Verification items for the finished model (mm, model axes). Round coordinates to 2 decimals unless told otherwise and drop trailing zeros. Order: outer loops, then holes, each group sorted by start corner. A loop starts at its lowest first (then second) coordinate and runs counter-clockwise, first axis right, second up. Notation, with made-up numbers: M -38.5,44.5 L 2.5,44.5 A20 ccw 2.5,74.5 Z; hole C -28,45.5 d9. An arc over 180 degrees is marked long. Use one line per item in the form item = value. Start each with the question number.
Item 1: Thickness scan on probe 1 along Y at (x, z) = (-61, 38.75); probe 2 along X at (y, z) = (-24.5, 45.25); probe 3 along Y at (x, z) = (-42, 39.5). Record the ranges inside material, lowest first. Write a range as [from, to].
Item 2: Release check for a two-part mould opening along X. For faces 1 (the flat face through (-12, 0, 42)), 2 (the flat face through (64.994, -50, 42)), 3 (the cylindrical face through (-23.12, -98.48, 42.16)), 4 (the cylindrical face through (-56.414, -96.911, 42.164)) record: +X half, -X half, draft (parallel to the pull), parting line (faces both ways), or undercut.
Item 3: Cross-section at B-B on y = -21.5. Enter the section's corners in (x, z), then the cut area to 3 significant figures.
Item 4: Go/stop test with a flat-tipped pin: pin 1 Ø7.5 at (x, y) = (-62.3, -6.68) entering from +Z. Record where the tip stops, or that it passes through.
Item 5: Cross-section at C-C on x = -77. Enter the section's corners in (y, z), then the cut area to 3 significant figures.
Item 6: Cross-section at A-A on z = 41.5. Count the separate pieces of the cut face and the enclosed holes in it, then the cut area to 3 significant figures.
from build123d import *

# Parameters (mm, degrees)
F1_DEPTH = 25.4
F2_DEPTH = 75.9968
F3_R     = 3.356014
F4_DEPTH = 56.388


with BuildPart() as f1:
    # F0 (on Front) → F1 (new body)
    with BuildSketch(Plane.XZ):
        Polygon((64.99356, 48.242185), (-85.765576, 48.242185), (-86.065296, 36.253385), (64.99356, 36.253385), align=None)
    extrude(amount=F1_DEPTH)

    # F1_face (on face) → F2 (join)
    with BuildSketch(Plane(origin=(-10.460963, -25.4, 42.245801), x_dir=(1, 0, 0), z_dir=(0, -1, 0))):
        Polygon((-75.604333, -5.992416), (75.454523, -5.992416), (75.454523, 5.996384), (-75.304613, 5.996384), align=None)
    extrude(amount=F2_DEPTH)

    # F3 (on Top) → F4 (cut)
    with BuildSketch(Plane.XY):
        with Locations((-76.532871, -6.641844)):
            Circle(F3_R)
        with Locations((-62.301904, -6.680765)):
            Circle(F3_R)
        with Locations((-76.775998, -95.625482)):
            Circle(F3_R)
        with Locations((-59.514143, -95.625482)):
            Circle(F3_R)
        with Locations((-39.810318, -6.680765)):
            Circle(F3_R)
        with Locations((-21.883452, -6.680765)):
            Circle(F3_R)
        with Locations((-39.810318, -95.201291)):
            Circle(F3_R)
        with Locations((-22.395648, -95.201291)):
            Circle(F3_R)
        with Locations((34.714222, -6.680765)):
            Circle(F3_R)
        with Locations((55.078939, -6.680765)):
            Circle(F3_R)
        with Locations((55.078939, -23.347175)):
            Circle(F3_R)
        with Locations((35.766117, -23.347175)):
            Circle(F3_R)
    extrude(amount=F4_DEPTH, mode=Mode.SUBTRACT)


solid = f1.part
Output values:
q1.probe_1 = [-101.4, -98.63], [-92.62, -9.77], [-3.59, 0]
q1.probe_2 = [-85.84, 32.61], [38.92, 51.93], [58.23, 64.99]
q1.probe_3 = [-101.4, -97.74], [-92.66, -9.22], [-4.14, 0]
q2.face_1 = draft
q2.face_2 = +X half
q2.face_3 = undercut
q2.face_4 = undercut
q3.outline = M -86.07,36.25 L 32.96,36.25 L 32.96,48.24 L -85.77,48.24 Z; M 38.57,36.25 L 52.28,36.25 L 52.28,48.24 L 38.57,48.24 Z; M 57.88,36.25 L 64.99,36.25 L 64.99,48.24 L 57.88,48.24 Z
q3.area = 1,670 mm2
q4.pin_1 = 48.24
q5.outline = M -101.4,36.25 L -98.97,36.25 L -98.97,48.24 L -101.4,48.24 Z; M -92.28,36.25 L -9.97,36.25 L -9.97,48.24 L -92.28,48.24 Z; M -3.32,36.25 L 0,36.25 L 0,48.24 L -3.32,48.24 Z
q5.area = 1,060 mm2
q6.separate_pieces = 1
q6.enclosed_holes = 12
q6.area = 14,900 mm2
